Here's how the part is built. I have some questions about the finished solid (model axes, mm). A direction names the side the tool comes from. Give positions to 0.01 mm unless a question says otherwise; leave off trailing zeros. Loops run counter-clockwise (first coordinate to the right, second up) from the corner with the lowest first, then second, coordinate; pieces in that order, holes last. Notation, with made-up numbers: (-20, 30) - (9, 30) arc R31 ccw to (9, 63) - close; hole circle Ø3 at (25, 13). An arc over 180 degrees is marked (long way). Return JSON: item names as keys, results as strings. Group by question number.
(1) If we section it at B-B (x = 0): Please give me the cut outline in (y, z), then the cut area to 4 significant figures.
(2) If we section it at C-C (z = 13): Please give me the cut outline in (x, y), then the cut area to 3 significant figures.
(3) For P1, Ø3, axis at x = 1, z = 2.5, coming from the +Y side; P2, Ø4, axis at x = -7, z = 20.5, coming from the -Y side; P3, Ø4, axis at x = -9.5, y = 0, coming from the -Z side; P4, Ø4, axis at x = 9.5, y = 0, coming from the +Z side, each with a flat end and sliding along its axis, tell me the tip position at first contact or that it passes through.
(4) If we section it at A-A (y = 40): Please give me the cut outline in (x, z).
(5) On a 3-axis mill with a long thin cutter (end or side, diameter ignored), from which of +Z, -Z, +X, -X, +Y, -Y can I reach the whole of each face in a straight line? I mean faces 1 (the flat face through (0, 28, 2)), 2 (the flat face through (7.5, 33, 14)), 3 (the flat face through (0, 35, 8)), 4 (the flat face through (12, 28, 6)). Say none if no direction works.
(6) I need wall thicknesses on probe 1 along Y at (x, z) = (0, 2.65); probe 2 along Y at (x, z) = (8, 28.4); probe 3 along Y at (x, z) = (-12.5, 22). Which ranges of each line are inside material? Lowest first, please. Write a range as [from, to].
(7) If we section it at D-D (y = 4): Please give me the cut outline in (x, z), then the cut area to 3 significant figures.
(8) If we mould it in two halves opening along Z, with no side actions, what happens to faces 5 (the cylindrical face through (-8.325, 38.536, 27.528)), 6 (the flat face through (-7.5, 33, 14)), 7 (the flat face through (0, 44, 25.5))? For each: released by +Z, released by -Z, zero draft, split by the parting line, or undercut.
```python
from build123d import *

# Parameters (mm, degrees)
SKETCH_1_R          = 6.5
SKETCH_1_W          = 15
SKETCH_1_H          = 18
EXTRUDE_1_DEPTH     = 3.5
HOLE_WIZARD_M3_1_D  = 2.5
FILLET_1_R          = 3
SKETCH_2_W          = 26
SKETCH_2_H          = 4
EXTRUDE_2_DEPTH     = 30
SKETCH_4_R          = 1.5
EXTRUDE_3_DEPTH     = 4
CHAMFER_1_SIZE      = 2
SKETCH_5_W          = 15
SKETCH_5_H          = 8
CUT_EXTRUDE_1_DEPTH = 10
FILLET_2_R          = 2
EXTRUDE_4_DEPTH     = 3
EXTRUDE_5_DEPTH     = 3


with BuildPart() as part:
    # 草图1 → 凸台-拉伸1 (new body)
    with BuildSketch(Plane.XY):
        with BuildLine():
            Line((-15, 35), (15, 35))
            Line((15, 35), (15, 0))
            ThreePointArc((15, 0), (0, -15), (-15, 0))
            Line((-15, 0), (-15, 35))
        make_face()
        Circle(SKETCH_1_R, mode=Mode.SUBTRACT)
        with Locations((0, 19)):
            Rectangle(SKETCH_1_W, SKETCH_1_H, mode=Mode.SUBTRACT)
    extrude(amount=EXTRUDE_1_DEPTH)

    # M3 螺纹孔1 (through all)
    with Locations(Plane.XY.offset(3.5)):
        with Locations((9.5, 0), (-9.5, 0)):
            Hole(HOLE_WIZARD_M3_1_D / 2)

    # 圆角1
    fillet_1_edges = [part.edges().sort_by_distance(p)[0] for p in [
        (-7.5, 10, 1.75),
        (7.5, 10, 1.75),
        (7.5, 28, 1.75),
        (-7.5, 28, 1.75),
    ]]
    fillet(fillet_1_edges, radius=FILLET_1_R)

    # 草图2 → 凸台-拉伸2 (add, through all)
    with BuildSketch(Plane(origin=(15, 0, 0), x_dir=(0, 0, -1), z_dir=(1, 0, 0))):
        with Locations((-16.5, 33)):
            Rectangle(SKETCH_2_W, SKETCH_2_H)
    extrude(amount=-EXTRUDE_2_DEPTH)

    # 草图4 → 凸台-拉伸3 (add)
    with BuildSketch(Plane.XY.offset(29.5)):
        Polygon((-15, 35), (-6, 55), (6, 55), (15, 35), align=None)
        with Locations((0, 49)):
            Circle(SKETCH_4_R, mode=Mode.SUBTRACT)
        with Locations((-8, 40)):
            Circle(SKETCH_4_R, mode=Mode.SUBTRACT)
        with Locations(Location((8, 40, 0), (0, 0, 180))):
            Circle(SKETCH_4_R, mode=Mode.SUBTRACT)
    extrude(amount=-EXTRUDE_3_DEPTH)

    # 倒角1
    chamfer_1_edges = [part.edges().sort_by_distance(p)[0] for p in [
        (0, 35, 0),
        (0, 31, 3.5),
        (0, 31, 29.5),
        (0, 35, 25.5),
    ]]
    chamfer(chamfer_1_edges, length=CHAMFER_1_SIZE)

    # 草图5 → 切除-拉伸1 (cut)
    with BuildSketch(Plane(origin=(0, 35, 0), x_dir=(1, 0, 0), z_dir=(0, 1, 0))):
        with Locations((0, -14)):
            Rectangle(SKETCH_5_W, SKETCH_5_H)
    extrude(amount=-CUT_EXTRUDE_1_DEPTH, mode=Mode.SUBTRACT)

    # 圆角2
    fillet_2_edges = [part.edges().sort_by_distance(p)[0] for p in [
        (-7.5, 33, 18),
        (-7.5, 33, 10),
        (7.5, 33, 10),
        (7.5, 33, 18),
    ]]
    fillet(fillet_2_edges, radius=FILLET_2_R)

    # 草图6 → 凸台-拉伸4 (add)
    with BuildSketch(Plane.ZY.offset(15)):
        Polygon((3.5, 24), (10.5, 31), (5.5, 31), (3.5, 29), align=None)
    extrude(amount=-EXTRUDE_4_DEPTH)

    # 草图7 → 凸台-拉伸5 (add)
    with BuildSketch(Plane(origin=(15, 0, 0), x_dir=(0, 0, -1), z_dir=(1, 0, 0))):
        Polygon((-3.5, 24), (-3.5, 29), (-5.5, 31), (-10.5, 31), align=None)
    extrude(amount=-EXTRUDE_5_DEPTH)


solid = part.part
```
Values:
{
 "1": {"outline": "(-15, 0) - (-6.5, 0) - (-6.5, 3.5) - (-15, 3.5) - close; (6.5, 0) - (10, 0) - (10, 3.5) - (6.5, 3.5) - close; (28, 0) - (33, 0) - (35, 2) - (35, 10) - (31, 10) - (31, 5.5) - (29, 3.5) - (28, 3.5) - close; (31, 18) - (35, 18) - (35, 23.5) - (37, 25.5) - (47.5, 25.5) - (47.5, 29.5) - (33, 29.5) - (31, 27.5) - close; (50.5, 25.5) - (55, 25.5) - (55, 29.5) - (50.5, 29.5) - close", "area": "206.5 mm2"},
 "2": {"outline": "(-15, 31) - (-7.5, 31) - (-7.5, 35) - (-15, 35) - close; (7.5, 31) - (15, 31) - (15, 35) - (7.5, 35) - close", "area": "60.0 mm2"},
 "3": {"P1": "y = 35", "P2": "y = 31", "P3": "z = 0", "P4": "z = 3.5"},
 "4": {"outline": "(-12.75, 25.5) - (-9.5, 25.5) - (-9.5, 29.5) - (-12.75, 29.5) - close; (-6.5, 25.5) - (6.5, 25.5) - (6.5, 29.5) - (-6.5, 29.5) - close; (9.5, 25.5) - (12.75, 25.5) - (12.75, 29.5) - (9.5, 29.5) - close"},
 "5": {"face 1": "+Z, -Z", "face 2": "+Y, -Y", "face 3": "-Z, +X, -X, +Y", "face 4": "+Z, -Y"},
 "6": {"probe 1": "[-15, -6.5], [6.5, 10], [28, 35]", "probe 2": "[31.9, 38.5], [41.5, 50.56]", "probe 3": "[31, 35]"},
 "7": {"outline": "(-15, 0) - (-5.12, 0) - (-5.12, 3.5) - (-15, 3.5) - close; (5.12, 0) - (15, 0) - (15, 3.5) - (5.12, 3.5) - close", "area": "69.1 mm2"},
 "8": {"face 5": "zero draft", "face 6": "undercut", "face 7": "released by -Z"}
}
